Build history of the part. All positions in model axes, mm. Face numbers are marked on the shaded views. A direction names the side the tool comes from. Give positions to 0.01 mm unless a question says otherwise; leave off trailing zeros. Loops run counter-clockwise (first coordinate to the right, second up) from the corner with the lowest first, then second, coordinate; pieces in that order, holes last. Notation, with made-up numbers: (-7, -10) -> (1, -10) arc R28 cw to (1, 23) -> close; hole circle Ø2 at (40, 42.5). An arc over 180 degrees is marked (long way). Answer as a JSON object with one key per item and string values. Group by question number.
Q1. Drop flat-ended pins along their axis: pin 1 (3 mm diameter, centred on x = 2, y = 3.5, fed in from -Z); pin 2 (1 mm diameter, centred on x = 0.5, y = 5, fed in from -Z); pin 3 (0.8 mm diameter, centred on x = -0.5, z = 0, fed in from -Y). Give the stop position or say it passes through.
Q2. Two-plate mould, pull along X, no slides. Class the marked faces 4, 5 and 6: pulls with the +X half, pulls with the -X half, needs draft (parallel to the pull), parting line crosses it, or undercut.
Q3. Band-saw the part on A-A, the plane z = 0. Write the cut outline in (x, y).
Q4. Band-saw the part on B-B, the plane y = -2.5. Write the cut outline in (x, z).
Q5. Tool access for the marked faces 1, 2 and 3: list every direction of +Z, -Z, +X, -X, +Y, -Y with a clear straight run to the whole face (end or side of a thin tool).
Q6. Band-saw the part on C-C, the plane y = -0.75. Write the cut outline in (x, z).
Q7. Band-saw the part on D-D, the plane y = 4.75. Write the cut outline in (x, z), plus the area to 3 significant figures.
Q8. Wall check: probe 1 along Y at (x, z) = (-0.6, -0.1); probe 2 along Z at (x, y) = (0.1, 4.75). Give the ranges that are in metal, low to high. Write a range as from..to.
from build123d import *

# Parameters (mm, degrees)
F0_R     = 1.5
F1_DEPTH = 8
F0_R_2   = 2.5
F2_DEPTH = 4
F4_DEPTH = 2
F5_SIZE  = 0.4


# Not quite as in the source:
# - a feature names something its author has since deleted; it is built from what else it names


with BuildPart() as f1:
    # F0 (on Front) → F1 (new body)
    with BuildSketch(Plane.XZ):
        Circle(F0_R)
    extrude(amount=-F1_DEPTH)

    # F0 (on Front) → F2 (join)
    with BuildSketch(Plane.XZ):
        Circle(F0_R_2)
        Circle(F0_R, mode=Mode.SUBTRACT)
        Circle(F0_R)
    extrude(amount=F2_DEPTH)

    # F3 (on face) → F4 (cut)
    with BuildSketch(Plane.XZ.offset(4)):
        Polygon((1.25, -0.7216878365), (1.25, 0.7216878365), (0, 1.443375673), (-1.25, 0.7216878365), (-1.25, -0.7216878365), (0, -1.443375673), align=None)
    extrude(amount=-F4_DEPTH, mode=Mode.SUBTRACT)

    # F5
    f5_edges = [f1.edges().sort_by_distance(p)[0] for p in [
        (-2.5, -4, 0),
        (-1.5, 8, 0),
    ]]
    chamfer(f5_edges, length=F5_SIZE)


solid = f1.part
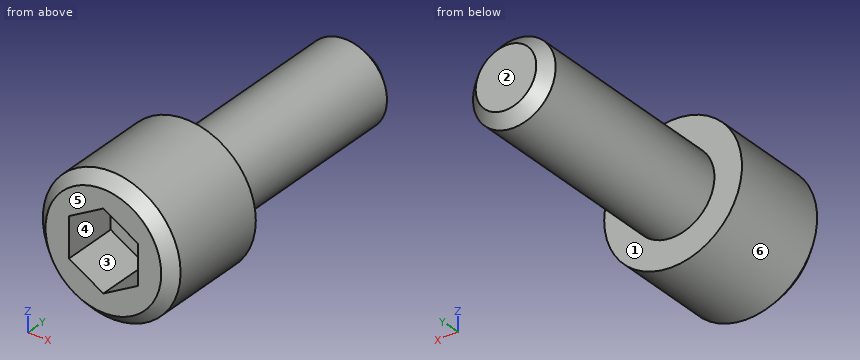
Worked answers:
{
 "1": {"pin 1": "z = -1.41", "pin 2": "z = -1.5", "pin 3": "y = -2"},
 "2": {"face 4": "undercut", "face 5": "needs draft", "face 6": "parting line crosses it"},
 "3": {"outline": "(-2.5, -3.6) -> (-2.1, -4) -> (-1.25, -4) -> (-1.25, -2) -> (1.25, -2) -> (1.25, -4) -> (2.1, -4) -> (2.5, -3.6) -> (2.5, 0) -> (1.5, 0) -> (1.5, 7.6) -> (1.1, 8) -> (-1.1, 8) -> (-1.5, 7.6) -> (-1.5, 0) -> (-2.5, 0) -> close"},
 "4": {"outline": "circle Ø5 at (0, 0); hole (-1.25, -0.72) -> (0, -1.44) -> (1.25, -0.72) -> (1.25, 0.72) -> (0, 1.44) -> (-1.25, 0.72) -> close"},
 "5": {"face 1": "+Y", "face 2": "+Z, -Z, +X, -X, +Y", "face 3": "-Y"},
 "6": {"outline": "circle Ø5 at (0, 0)"},
 "7": {"outline": "circle Ø3 at (0, 0)", "area": "7.07 mm2"},
 "8": {"probe 1": "-2..8", "probe 2": "-1.5..1.5"}
}
